Here's how the part is built. I have some questions about the finished solid (model axes, mm). Face numbers are marked on the shaded views. A direction names the side the tool comes from. Coordinates: 2 decimals unless noted, no trailing zeros. Order: outer loops, then holes, each group sorted by start corner. A loop starts at its lowest first (then second) coordinate and runs counter-clockwise, first axis right, second up. Notation, with made-up numbers: M -21,75 L -1,75 A24 ccw -1,110 Z; hole C 11.5,-25 d10. An arc over 180 degrees is marked long. Answer as CSV lines item,"result". Start each with the question number.
```python
from build123d import *

# Parameters (mm, degrees)
F0_W     = 645
F0_H     = 413
F0_W_2   = 633
F0_H_2   = 401
F1_DEPTH = 400
F2_W     = 645
F2_H     = 413
F3_DEPTH = 6


with BuildPart() as f1:
    # F0 (on Top) → F1 (new body)
    with BuildSketch(Plane.XY):
        Rectangle(F0_W, F0_H)
        Rectangle(F0_W_2, F0_H_2, mode=Mode.SUBTRACT)
    extrude(amount=-F1_DEPTH)

    # F2 (on face) → F3 (join)
    with BuildSketch(Plane(origin=(0, 0, -400), x_dir=(1, 0, 0), z_dir=(0, 0, -1))):
        Rectangle(F2_W, F2_H)
    extrude(amount=F3_DEPTH)


solid = f1.part
```
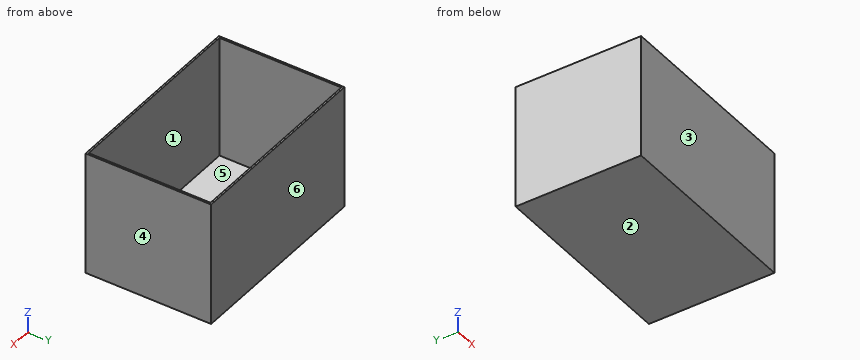
1) Which directions (+Z, -Z, +X, -X, +Y, -Y) give clear straight access to the entire face, cutting with the end or side of a thin tool? Please do the marked faces 1 and 2.
2) If we mould it in two halves opening along Y, with no side actions, what happens to the marked faces 3, 4, 5 and 6? For each: released by +Y, released by -Y, zero draft, split by the parting line, or undercut.
3) Suppose I cut it at A-A on z = -294. Please give me the cut outline in (x, y), plus the area to 3 significant figures.
4) Will this pin go through, and if not, where does the flat tip stop? pin 1 Ø2 at (x, y) = (-159, -61.5) entering from +Z.
5) Suppose I cut it at B-B on x = 102.5. Please give me the cut outline in (y, z), plus the area to 3 significant figures.
6) I need wall thicknesses on line 1 (X direction, y = 187.5, z = -298); line 2 (Y direction, x = -11, z = -70); line 3 (Z direction, x = 266, y = -129). Which ranges of each line are inside material? Lowest first, please. Write a range as [from, to].
7) Suppose I cut it at C-C on y = 121. Please give me the cut outline in (x, z), plus the area to 3 significant figures.
Output:
1,face 1,"+Z"
1,face 2,"-Z, +X, -X, +Y, -Y"
2,face 3,"released by -Y"
2,face 4,"zero draft"
2,face 5,"undercut"
2,face 6,"released by +Y"
3,outline,"M -322.5,-206.5 L 322.5,-206.5 L 322.5,206.5 L -322.5,206.5 Z; hole M -316.5,-200.5 L 316.5,-200.5 L 316.5,200.5 L -316.5,200.5 Z"
3,area,"12,600 mm²"
4,pin 1,"z = -400"
5,outline,"M -206.5,-406 L 206.5,-406 L 206.5,0 L 200.5,0 L 200.5,-400 L -200.5,-400 L -200.5,0 L -206.5,0 Z"
5,area,"7,280 mm²"
6,line 1,"[-322.5, -316.5], [316.5, 322.5]"
6,line 2,"[-206.5, -200.5], [200.5, 206.5]"
6,line 3,"[-406, -400]"
7,outline,"M -322.5,-406 L 322.5,-406 L 322.5,0 L 316.5,0 L 316.5,-400 L -316.5,-400 L -316.5,0 L -322.5,0 Z"
7,area,"8,670 mm²"
